Autodesk Inventor part; units mm, degrees
ref_plane "YZ Plane" through (0, 0, 0) normal (1, 0, 0) x (0, 1, 0)
ref_plane "XZ Plane" through (0, 0, 0) normal (0, 1, 0) x (-1, 0, 0)
ref_plane "XY Plane" through (0, 0, 0) normal (0, 0, 1) x (1, 0, 0)
sketch "Sketch1" plane through (0, 0, 0) normal (0, 1, 0) x (-1, 0, 0)
  line L0 (-1, 9) -> (1, 9)
  line L1 (1, 9) -> (1, -9)
  line L2 (1, -9) -> (-1, -9)
  line L3 (-1, -9) -> (-1, 9)
  line L4 (-1, 9) -> (1, -9) construction
  line L5 (1, 9) -> (-1, -9) construction
  point P0 (0, 0)
  dimension "d0" = 18
  dimension "d1" = 2
extrude "Extrusion1" add sketch "Sketch1" along normal blind 8
fillet "Fillet1" radius 2 2 edges at (0, 8, 9) (0, 8, -9)
sketch "Sketch2" plane through (1, 0, 9) normal (1, 0, 0) x (0, 0, -1)
  circle A0 centre (2.5, 5.5) radius 1.2
  circle A1 centre (15.5, 5.5) radius 1.2
  line L0 (2, 8) -> (16, 8)
  line L1 (18, 0) -> (18, 6)
  line L2 (0, 0) -> (0, 6)
  point P0 (9, 0)
  point P1 (0, 3)
  dimension "d5" = 2.4
  dimension "d6" = 2.4
  dimension "d7" = 2.5
  dimension "d8" = 2.5
  dimension "d9" = 2.5
  dimension "d10" = 2.5
extrude "Extrusion2" cut sketch "Sketch2" against normal blind 2
fillet "Fillet2" radius 2 2 edges at (0, 0, 9) (0, 0, -9)
sketch "Sketch5" plane through (1, 8, 7) normal (1, 0, 0) x (0, 0, -1)
  line L0 (5.5, -8) -> (8.5, -8)
  line L1 (8.5, -8) -> (8.5, 0)
  line L2 (8.5, 0) -> (5.5, 0)
  line L3 (5.5, 0) -> (5.5, -8)
  line L4 (5.5, -8) -> (8.5, 0) construction
  line L5 (8.5, -8) -> (5.5, 0) construction
  line L6 (0, 0) -> (14, 0)
  line L7 (0, -8) -> (14, -8)
  line L8 (7, 0) -> (7, -8) construction
  line L9 (-2, -6) -> (-2, -2)
  line L10 (-2, -4) -> (16, -4) construction
  line L11 (16, -6) -> (16, -2)
  point P0 (7, -4)
  dimension "d14" = 3
extrude "Extrusion3" add sketch "Sketch5" along normal blind 10
fillet "Face Fillet1" radius 2 1 edges at (1, 4, 1.5)
fillet "Face Fillet2" radius 2 1 edges at (1, 4, -1.5)
properties part number "Uchwyt"
Input: part model. Units: mm. Frame: model coordinates. A direction names the side the tool comes from. Give positions to 0.01 mm unless a question says otherwise; leave off trailing zeros. Order: outer loops, then holes, each group sorted by start corner. A loop starts at its lowest first (then second) coordinate and runs counter-clockwise, first axis right, second up.
Q1. Set-up query: faces 1 (the cylindrical face through (-0.01, 0.57, 8.4)), 2 (the flat face through (7, 4, -1.5)), 3 (the flat face through (1, 4, 6)). Return all of +Z, -Z, +X, -X, +Y, -Y with unobstructed straight access to the full face (end or side cutting, diameter ignored); none if empty.
Checked values:
face 1: +Z, +X, -X, -Y
face 2: -Z, +X, +Y, -Y
face 3: +Z, +X, +Y, -Y
Q2. Section C-C on x = 0.5. Output: boundary loops of the cut face in (y, z), and give its area (3 significant figures).
Checked values:
outline: (0, -7) arc R2 ccw to (2, -9) - (6, -9) arc R2 ccw to (8, -7) - (8, 7) arc R2 ccw to (6, 9) - (2, 9) arc R2 ccw to (0, 7) - close; hole circle Ø2.4 at (5.5, -6.5); hole circle Ø2.4 at (5.5, 6.5)
area: 132 mm2
Q3. Contact query for flat-ended pins moving along their axis: pin 1 Ø2 at (y, z) = (5.5, -6.5) entering from +X; pin 2 Ø2.5 at (x, y) = (5.5, 3) entering from -Z; pin 3 Ø4 at (x, y) = (5, 2.5) entering from +Z. Output: stop coordinate, or through.
Checked values:
pin 1: passes through
pin 2: stops at z = -1.5
pin 3: stops at z = 1.5
Q4. Section D-D on y = 3.5. Output: boundary loops of the cut face in (x, z).
Checked values:
outline: (-1, -9) - (1, -9) - (1, -3.5) arc R2 cw to (3, -1.5) - (11, -1.5) - (11, 1.5) - (3, 1.5) arc R2 cw to (1, 3.5) - (1, 9) - (-1, 9) - close
Q5. Ray query, probe 1 along Y at (x, z) = (-0.05, -6.5); probe 2 along Z at (x, y) = (7.5, 6.75); probe 3 along X at (y, z) = (3.25, -5.5). Return the intervals inside material, ascending.
Checked values:
probe 1: y = 0 to 4.3, 6.7 to 8
probe 2: z = -1.5 to 1.5
probe 3: x = -1 to 1
Q6. Section A-A on y = 5.5. Output: boundary loops of the cut face in (x, z).
Checked values:
outline: (-1, -9) - (1, -9) - (1, -7.7) - (-1, -7.7) - close; (-1, -5.3) - (1, -5.3) - (1, -3.5) arc R2 cw to (3, -1.5) - (11, -1.5) - (11, 1.5) - (3, 1.5) arc R2 cw to (1, 3.5) - (1, 5.3) - (-1, 5.3) - close; (-1, 7.7) - (1, 7.7) - (1, 9) - (-1, 9) - close
Q7. Draft query along Z for faces 4 (the cylindrical face through (0.01, 5.55, 7.7)), 5 (the cylindrical face through (1.57, 4.06, -2.1)), 6 (the cylindrical face through (0.01, 5.55, -5.3)), 7 (the flat face through (7, 4, 1.5)). Return one class per face: +Z half, -Z half, draft (parallel to the pull), parting line (faces both ways), or undercut.
Checked values:
face 4: undercut
face 5: -Z half
face 6: undercut
face 7: +Z half
Q8. Section B-B on z = 6.5. Output: boundary loops of the cut face in (x, y).
Checked values:
outline: (-1, 0) - (1, 0) - (1, 4.3) - (-1, 4.3) - close; (-1, 6.7) - (1, 6.7) - (1, 8) - (-1, 8) - close
